For this review, take the finished solid that the model builds, in its own axes (mm). A direction names the side the tool comes from. Round coordinates to 2 decimals unless told otherwise and drop trailing zeros. Order: outer loops, then holes, each group sorted by start corner. A loop starts at its lowest first (then second) coordinate and runs counter-clockwise, first axis right, second up. Notation, with made-up numbers: M 56.5,-31.5 L 103.5,-31.5 A22 ccw 103.5,-2.5 Z; hole C 13,-38.5 d6. An arc over 180 degrees is marked long. Write item = value, one per line. Start each with the question number.
from build123d import *

# Parameters (mm, degrees)
SKETCH1_W           = 333.375
SKETCH1_H           = 285.75
SKETCH1_W_2         = 317.5
SKETCH1_H_2         = 269.875
BOSS_EXTRUDE1_DEPTH = 92.075
SKETCH2_R           = 2.54
CUT_EXTRUDE1_DEPTH  = 369.90049146
SKETCH3_R           = 3.175
CUT_EXTRUDE2_DEPTH  = 7.9375
SKETCH4_R           = 3.175
CUT_EXTRUDE3_DEPTH  = 7.9375


with BuildPart() as part:
    # Sketch1 → Boss-Extrude1 (new body)
    with BuildSketch(Plane(origin=(0, 0, 0), x_dir=(1, 0, 0), z_dir=(0, 1, 0))):
        with Locations((47.68764892, -69.90555659)):
            Rectangle(SKETCH1_W, SKETCH1_H)
        with Locations((47.68764892, -69.90555659)):
            Rectangle(SKETCH1_W_2, SKETCH1_H_2, mode=Mode.SUBTRACT)
    extrude(amount=BOSS_EXTRUDE1_DEPTH)

    # Sketch2 → Cut-Extrude1 (cut, through all)
    with BuildSketch(Plane.XY.offset(212.78055659)):
        with Locations((47.68764892, 79.375)):
            Circle(SKETCH2_R)
    extrude(amount=-CUT_EXTRUDE1_DEPTH, mode=Mode.SUBTRACT)

    # Sketch3 → Cut-Extrude2 (cut)
    with BuildSketch(Plane.XY.offset(212.78055659)):
        with Locations((47.68764892, 46.0375)):
            Circle(SKETCH3_R)
    extrude(amount=-CUT_EXTRUDE2_DEPTH, mode=Mode.SUBTRACT)

    # Sketch4 → Cut-Extrude3 (cut)
    with BuildSketch(Plane(origin=(214.37514892, 0, 0), x_dir=(0, 0, -1), z_dir=(1, 0, 0))):
        with Locations((-69.90555659, 38.559584582)):
            Circle(SKETCH4_R)
    extrude(amount=-CUT_EXTRUDE3_DEPTH, mode=Mode.SUBTRACT)


solid = part.part
(1) We need section C-C, the plane y = 9.5. Write out the cut boundary in (x, z).
(2) For faces 1 (the flat face through (35, 0, 207)), 2 (the flat face through (45, 35, 204.843)), list the 3-axis set-ups (+Z, -Z, +X, -X, +Y, -Y) from which the entire face can be reached by the end or side of a thin tool; tool diameter is ignored.
(3) For line 1 along Z through (x, y) = (-17.5, 53); line 2 along X through (y, z) = (80, -47), list the stretches that pass through material, from the lowest coordinate up.
(4) Draft analysis for pull direction Z (two halves, no side actions). For faces 3 (the flat face through (-111.062, 45, 72)), 4 (the flat face through (45, 45, -72.969)), 5 (the flat face through (-119, 45, 72)), state which applies: released by +Z, released by -Z, zero draft, split by the parting line, or undercut.
(5) Insertion check: pin 1 (4 mm diameter, centred on x = 47.69, y = 79.38, fed in from +Z). The pin has a flat end and moves straight along its axis. Give the tip position at first contact, or say it passes through.
(6) We need section B-B, the plane x = 178. Write out the cut boundary in (y, z) (3 decimals), then the cut area to 3 significant figures.
(7) We need section A-A, the plane z = 107.5. Write out the cut boundary in (x, y) (3 decimals), then the cut area to 3 significant figures.
Values:
q1.outline = M -119,-72.97 L 214.38,-72.97 L 214.38,212.78 L -119,212.78 Z; hole M -111.06,-65.03 L 206.44,-65.03 L 206.44,204.84 L -111.06,204.84 Z
q2.face_1 = +Z, -Z, +X, -X, -Y
q2.face_2 = +Y, -Y
q3.line_1 = -72.97 to -65.03, 204.84 to 212.78
q3.line_2 = -119 to -111.06, 206.44 to 214.38
q4.face_3 = undercut
q4.face_4 = released by -Z
q4.face_5 = zero draft
q5.pin_1 = through
q6.outline = M 0,-72.969 L 92.075,-72.969 L 92.075,-65.032 L 0,-65.032 Z; M 0,204.843 L 92.075,204.843 L 92.075,212.781 L 0,212.781 Z
q6.area = 1,460 mm²
q7.outline = M -119,0 L -111.062,0 L -111.062,92.075 L -119,92.075 Z; M 206.438,0 L 214.375,0 L 214.375,92.075 L 206.438,92.075 Z
q7.area = 1,460 mm²
